Job drawing, mm, ordinate dimensions from the low corner. One solid piece. A direction names the side the tool comes from. Give positions to 0.01 mm unless a question says otherwise; leave off trailing zeros. Order: outer loops, then holes, each group sorted by start corner. A loop starts at its lowest first (then second) coordinate and runs counter-clockwise, first axis right, second up.
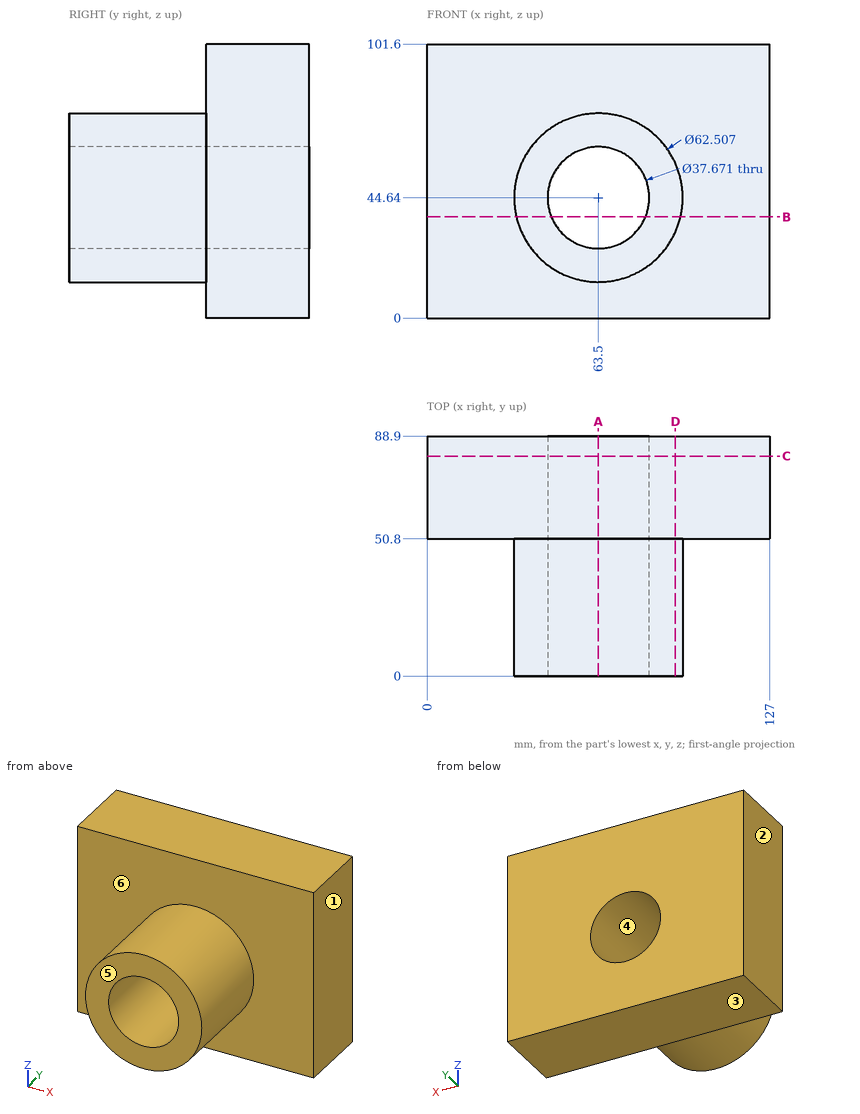
Item 1: Pull direction X, two halves, no side cores. Call the marked faces 1, 2, 3 and 4: released by +X, released by -X, zero draft, split by the parting line, or undercut.
Item 2: Drop flat-ended pins along their axis: P1, Ø8, axis at y = 23, z = 63, coming from the +X side; P2, Ø1, axis at y = 25, z = 49, coming from the +X side (1 decimal); P3, Ø5, axis at x = 51.5, y = 44, coming from the +Z side (1 decimal). Give the stop position or say it passes through.
Item 3: Band-saw the part on B-B on z = 37.5. List the corners of the cut face in (x, y), plus the area to 3 significant figures.
Item 4: Band-saw the part on D-D on x = 92. List the corners of the cut face in (y, z).
Item 5: Which spindle directions (+Z, -Z, +X, -X, +Y, -Y) get a long thin tool onto all of the face, cutting with end or side? Do the marked faces 5 and 6. Say none if no direction does.
Item 6: Drill centre lines: probe 1 along Z at (x, y) = (63.5, 22) (1 decimal); probe 2 along Z at (x, y) = (63, 65); probe 3 along Y at (x, z) = (18, 25). Where is each one in solid material? Low to high.
Item 7: Band-saw the part on A-A on x = 63.5. List the corners of the cut face in (y, z) (1 decimal), plus the area to 3 significant figures.
Item 8: Band-saw the part on C-C on y = 81.5. List the corners of the cut face in (x, z) (1 decimal).
Working result:
1. face 1: released by +X
1. face 2: released by -X
1. face 3: zero draft
1. face 4: undercut
2. P1: stops at x = 91.26
2. P2: stops at x = 94.5
2. P3: stops at z = 74.4
3. outline: (0, 50.8) - (33.07, 50.8) - (33.07, 0) - (46.07, 0) - (46.07, 88.9) - (0, 88.9) - close; (80.93, 0) - (93.93, 0) - (93.93, 50.8) - (127, 50.8) - (127, 88.9) - (80.93, 88.9) - close
3. area: 4,830 mm2
4. outline: (0, 31.81) - (50.8, 31.81) - (50.8, 0) - (88.9, 0) - (88.9, 101.6) - (50.8, 101.6) - (50.8, 57.47) - (0, 57.47) - close
5. face 5: +Z, -Z, +X, -X, -Y
5. face 6: -Y
6. probe 1: z = 13.4 to 25.8, 63.5 to 75.9
6. probe 2: z = 0 to 25.81, 63.47 to 101.6
6. probe 3: y = 50.8 to 88.9
7. outline: (0, 13.4) - (50.8, 13.4) - (50.8, 0) - (88.9, 0) - (88.9, 25.8) - (0, 25.8) - close; (0, 63.5) - (88.9, 63.5) - (88.9, 101.6) - (50.8, 101.6) - (50.8, 75.9) - (0, 75.9) - close
7. area: 3,700 mm2
8. outline: (0, 0) - (127, 0) - (127, 101.6) - (0, 101.6) - close; hole circle Ø37.7 at (63.5, 44.6)
